```python
from build123d import *

# Parameters (mm, degrees)
SKETCH1_W           = 25.4
SKETCH1_H           = 25.4
BOSS_EXTRUDE1_DEPTH = 25.4
SKETCH2_W           = 22.225
SKETCH2_H           = 22.225
CUT_EXTRUDE1_DEPTH  = 44.994090512
CUT_EXTRUDE2_DEPTH  = 44.994090512
HOLE1_D             = 8.3312
FILLET1_R           = 2.3622
FILLET2_R           = 3.175


with BuildPart() as part:
    # Sketch1 → Boss-Extrude1 (new body)
    with BuildSketch(Plane(origin=(0, 0, 0), x_dir=(0, 0, -1), z_dir=(1, 0, 0))):
        with Locations((-12.7, -12.7)):
            Rectangle(SKETCH1_W, SKETCH1_H)
    extrude(amount=-BOSS_EXTRUDE1_DEPTH)

    # Sketch2 → Cut-Extrude1 (cut, through all)
    with BuildSketch(Plane.XZ.offset(25.4)):
        with Locations((-14.2875, 14.2875)):
            Rectangle(SKETCH2_W, SKETCH2_H)
    extrude(amount=-CUT_EXTRUDE1_DEPTH, mode=Mode.SUBTRACT)

    # Sketch3 → Cut-Extrude2 (cut, through all)
    with BuildSketch(Plane(origin=(0, 0, 0), x_dir=(0, 0, -1), z_dir=(1, 0, 0))):
        with BuildLine():
            Line((-18.2626, -16.8656), (-11.9126, -16.8656))
            ThreePointArc((-11.9126, -16.8656), (-7.747, -12.7), (-11.9126, -8.5344))
            Line((-11.9126, -8.5344), (-18.2626, -8.5344))
            ThreePointArc((-18.2626, -8.5344), (-22.4282, -12.7), (-18.2626, -16.8656))
        make_face()
    extrude(amount=-CUT_EXTRUDE2_DEPTH, mode=Mode.SUBTRACT)

    # Hole1 (through all)
    with Locations(Plane.XY.offset(3.175)):
        with Locations((-12.7, -12.7)):
            Hole(HOLE1_D / 2)

    # Fillet1
    fillet1_edges = [part.edges().sort_by_distance(p)[0] for p in [
        (-25.4, -12.7, 3.175),
        (-3.175, -12.7, 25.4),
    ]]
    fillet(fillet1_edges, radius=FILLET1_R)

    # Fillet2
    fillet2_edges = [part.edges().sort_by_distance(p)[0] for p in [
        (-3.175, -12.7, 3.175),
    ]]
    fillet(fillet2_edges, radius=FILLET2_R)


solid = part.part
```
Geometry check sheet. Reference: the model listing, model coordinates, mm. A direction names the side the tool comes from. Coordinates: 2 decimals unless noted, no trailing zeros. Order: outer loops, then holes, each group sorted by start corner. A loop starts at its lowest first (then second) coordinate and runs counter-clockwise, first axis right, second up. Notation, with made-up numbers: (39.25, 71) - (84.25, 71) arc R24 ccw to (84.25, 99) - close; hole circle Ø4 at (77.5, 67.25). An arc over 180 degrees is marked (long way). Answer as a JSON object with one key per item and string values. Group by question number.
Item 1: Sectioned sample at D-D, the plane y = -7. Record the cut outline in (x, z) (3 decimals).
Item 2: Draft check along Y on faces 4 (the face through (-3, 0, 5)), 5 (the face through (-7, -13, 0)), 6 (the face through (-3, -25.4, 5)), 7 (the face through (-1.565, -12.608, 22.427)). Enter one of: +Y half, -Y half, draft (parallel to the pull), parting line (faces both ways), or undercut.
Item 3: Depth check by flat-ended pin: pin 1 Ø5 at (y, z) = (-3.5, 4) entering from -X; pin 2 Ø13.5 at (y, z) = (-13.5, 16.5) entering from -X (3 decimals); pin 3 Ø8 at (x, y) = (-22.5, -11.5) entering from +Z (3 decimals). Enter the tip coordinate at first touch or a pass-through.
Item 4: Scan lines: probe 1 along Y at (x, z) = (-12.7, 1.6); probe 2 along Z at (x, y) = (-12.75, -7.25) (3 decimals); probe 3 along X at (y, z) = (-24, 18.75) (3 decimals). Record each from-to range of solid material in increasing order.
Item 5: Sectioned sample at A-A, the plane z = 16.5. Record the cut outline in (x, y) (3 decimals), and give its area (3 significant figures).
Item 6: Tool access check on faces 1 (the face through (-2, -8.534, 15)), 2 (the face through (-25.4, -12.5, 0.4)), 3 (the face through (-3.175, -19, 15)). Record the directions out of +Z, -Z, +X, -X, +Y, -Y that give a thin tool (end or side, any length) a straight path to the whole face; none if there is none.
Item 7: Sectioned sample at C-C, the plane y = -12.7. Record the cut outline in (x, z) (3 decimals).
Item 8: Sectioned sample at B-B, the plane x = -12.7. Record the cut outline in (y, z) (3 decimals).
Resolved:
{
 "1": {"outline": "(-25.4, 0) - (0, 0) - (0, 25.4) - (-0.813, 25.4) arc R2.362 ccw to (-3.175, 23.038) - (-3.175, 6.35) arc R3.175 cw to (-6.35, 3.175) - (-23.038, 3.175) arc R2.362 ccw to (-25.4, 0.813) - close"},
 "2": {"face 4": "+Y half", "face 5": "draft", "face 6": "-Y half", "face 7": "undercut"},
 "3": {"pin 1": "x = -25.3", "pin 2": "x = -3.175", "pin 3": "z = 3.175"},
 "4": {"probe 1": "-25.4 to -16.87, -8.53 to 0", "probe 2": "0 to 3.175", "probe 3": "-3.175 to 0"},
 "5": {"outline": "(-3.175, -25.4) - (0, -25.4) - (0, -16.866) - (-3.175, -16.866) - close; (-3.175, -8.534) - (0, -8.534) - (0, 0) - (-3.175, 0) - close", "area": "54.2 mm^2"},
 "6": {"face 1": "+X, -X", "face 2": "+Z, -Z, -X, +Y, -Y", "face 3": "+Z, -X, +Y, -Y"},
 "7": {"outline": "(-25.4, 0) - (-16.866, 0) - (-16.866, 3.175) - (-23.038, 3.175) arc R2.362 ccw to (-25.4, 0.813) - close; (-8.534, 0) - (0, 0) - (0, 7.747) - (-3.175, 7.747) - (-3.175, 6.35) arc R3.175 cw to (-6.35, 3.175) - (-8.534, 3.175) - close; (-3.175, 22.428) - (0, 22.428) - (0, 25.4) - (-0.813, 25.4) arc R2.362 ccw to (-3.175, 23.038) - close"},
 "8": {"outline": "(-25.4, 0) - (-16.866, 0) - (-16.866, 3.175) - (-25.4, 3.175) - close; (-8.534, 0) - (0, 0) - (0, 3.175) - (-8.534, 3.175) - close"}
}
